Geometry: see drawing. Coordinates: mm, zero at the bounding-box minimum. A direction names the side the tool comes from. Give positions to 0.01 mm unless a question says otherwise; leave off trailing zeros. Write each loop counter-clockwise with the first axis right and the second up, starting at its lowest first coordinate (ties: lowest second). Pieces come first, ordered by that corner, then holes. Notation, with made-up numbers: M 42.5,-20 L 86.5,-20 A17 cw 86.5,11 Z; hole C 83.25,-16.5 d11. An arc over 180 degrees is marked long. Use a Markdown table: item, result. Add a question column.
(1) Cut plane A-A (x = 17.5). Output: boundary loops of the cut face in (y, z), plus the area to 3 significant figures.
(2) Cut plane C-C (z = 58). Output: boundary loops of the cut face in (x, y).
(3) Cut plane B-B (y = 17.5). Output: boundary loops of the cut face in (x, z), plus the area to 3 significant figures.
(4) Cut plane D-D (x = 31). Output: boundary loops of the cut face in (y, z), plus the area to 3 significant figures.
(5) Draft query along Z for the marked faces 1, 2 and 3. Return one class per face: released by +Z, released by -Z, zero draft, split by the parting line, or undercut.
(6) Pin query (flat end, axial travel): pin 1 Ø4 at (y, z) = (14.5, 33.5) entering from -X; pin 2 Ø3 at (x, y) = (28.5, 4.5) entering from +Z; pin 3 Ø3 at (y, z) = (23.5, 26.5) entering from +X; pin 4 Ø1.8 at (x, y) = (26.5, 18.5) entering from -Z. Return the tip coordinate at first contact, or that it passes through.
(7) Reachability of the marked faces 4 and 5 from +Z, -Z, +X, -X, +Y, -Y: full face, straight path, thin tool, end or side. Return the list, or none.
(8) Material intervals for L1, parallel to Z at x = 34, y = 20.5; L2, parallel to X at y = 17, z = 28, sorted ascending.
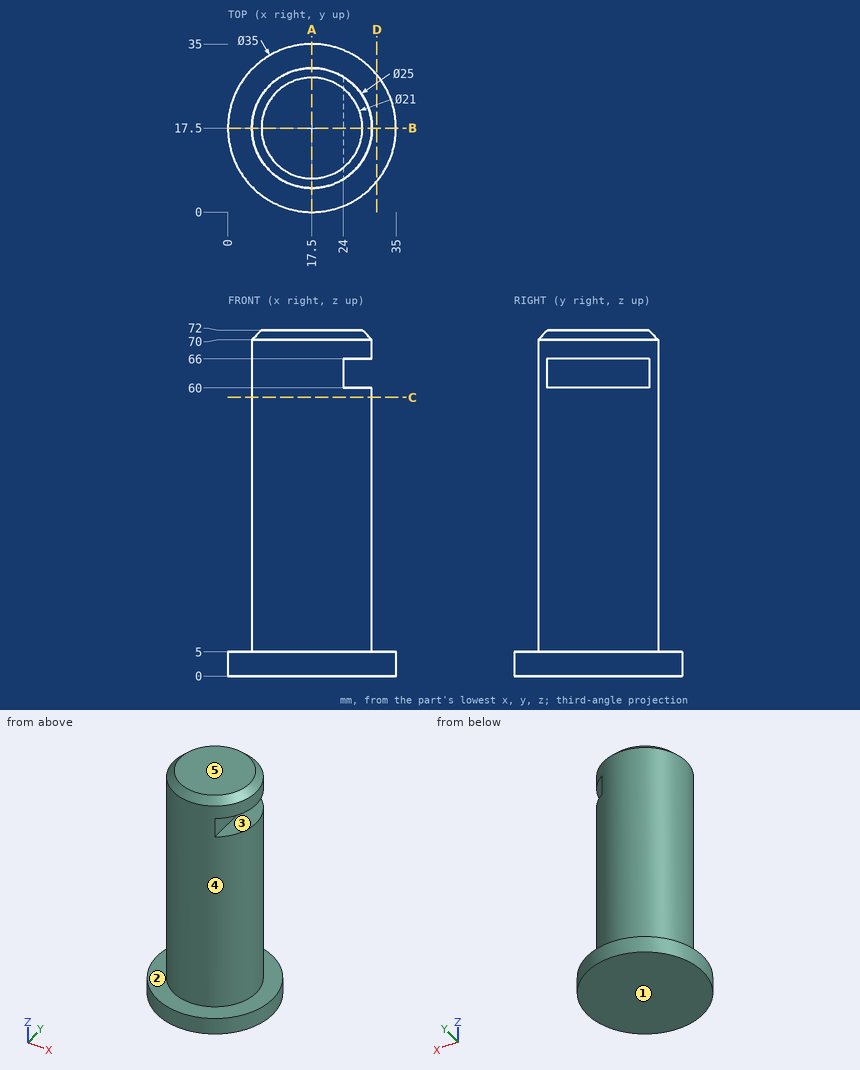
Answer list:
| question | item | result |
|---|---|---|
| 1 | outline | M 0,0 L 35,0 L 35,5 L 30,5 L 30,70 L 28,72 L 7,72 L 5,70 L 5,5 L 0,5 Z |
| 1 | area | 1,850 mm² |
| 2 | outline | C 17.5,17.5 d25 |
| 3 | outline | M 0,0 L 35,0 L 35,5 L 30,5 L 30,60 L 24,60 L 24,66 L 30,66 L 30,70 L 28,72 L 7,72 L 5,70 L 5,5 L 0,5 Z |
| 3 | area | 1,810 mm² |
| 4 | outline | M 6.36,0 L 28.64,0 L 28.64,5 L 6.36,5 Z |
| 4 | area | 111 mm² |
| 5 | face 1 | released by -Z |
| 5 | face 2 | released by +Z |
| 5 | face 3 | undercut |
| 6 | pin 1 | x = 5.04 |
| 6 | pin 2 | z = 5 |
| 6 | pin 3 | x = 29.16 |
| 6 | pin 4 | z = 0 |
| 7 | face 4 | +Z |
| 7 | face 5 | +Z, +X, -X, +Y, -Y |
| 8 | L1 | 0 to 5 |
| 8 | L2 | 5.01 to 29.99 |
